from build123d import *

# Parameters (mm, degrees)
ESBO_O1_W                = 20
ESBO_O1_H                = 28
ESBO_O1_R                = 1.5
RESSALTO_EXTRUS_O1_DEPTH = 6
ESBO_O2_W                = 5
ESBO_O2_H                = 12
RESSALTO_EXTRUS_O2_START = -29
ESBO_O3_W                = 20
ESBO_O3_H                = 20
RESSALTO_EXTRUS_O2_DEPTH = 10
CORTE_EXTRUS_O1_DEPTH    = 28


with BuildPart() as part:
    # Esboço1 → Ressalto-extrusão1 (new body, symmetric)
    with BuildSketch(Plane.XY):
        Rectangle(ESBO_O1_W, ESBO_O1_H)
        with Locations((-7, 10)):
            Circle(ESBO_O1_R, mode=Mode.SUBTRACT)
        with Locations((7, 10)):
            Circle(ESBO_O1_R, mode=Mode.SUBTRACT)
    extrude(amount=RESSALTO_EXTRUS_O1_DEPTH, both=True)

    # Esboço2 → Revolução1 (revolve)
    with BuildSketch(Plane.XY):
        Polygon((3, -29), (3, -19), (3, -14), (0, -14), (0, -34), (0.75, -34), (3.5, -32), (3.5, -29), align=None)
        with Locations((2.5, 20)):
            Rectangle(ESBO_O2_W, ESBO_O2_H)
    revolve(axis=Axis((0, 0, 0), (0, -1, 0)))

    # Esboço3 → Ressalto-extrusão2 (add)
    with BuildSketch(Plane(origin=(0, 0, 0), x_dir=(1, 0, 0), z_dir=(0, 1, 0)).offset(RESSALTO_EXTRUS_O2_START)):
        with Locations((0, 4)):
            Rectangle(ESBO_O3_W, ESBO_O3_H)
    extrude(amount=RESSALTO_EXTRUS_O2_DEPTH)

    # Esboço4 → Corte-extrusão1 (cut)
    with BuildSketch(Plane(origin=(0, 14, 0), x_dir=(1, 0, 0), z_dir=(0, 1, 0))):
        with BuildLine():
            ThreePointArc((-10, 0), (-9.486832981, 3.16227766), (-8, 6))
            Line((-8, 6), (-10, 6))
            Line((-10, 6), (-10, 0))
        make_face()
        with BuildLine():
            ThreePointArc((-8, -6), (-9.486832981, -3.16227766), (-10, 0))
            Line((-10, 0), (-10, -6))
            Line((-10, -6), (-8, -6))
        make_face()
        with BuildLine():
            Line((10, -6), (10, 0))
            ThreePointArc((10, 0), (9.486832981, -3.16227766), (8, -6))
            Line((8, -6), (10, -6))
        make_face()
        with BuildLine():
            Line((10, 6), (8, 6))
            ThreePointArc((8, 6), (9.486832981, 3.16227766), (10, 0))
            Line((10, 0), (10, 6))
        make_face()
    extrude(amount=-CORTE_EXTRUS_O1_DEPTH, mode=Mode.SUBTRACT)


solid = part.part
Work out the finished part from the listing and answer in its coordinate system (mm). A direction names the side the tool comes from. Give positions to 0.01 mm unless a question says otherwise; leave off trailing zeros. Order: outer loops, then holes, each group sorted by start corner. A loop starts at its lowest first (then second) coordinate and runs counter-clockwise, first axis right, second up. Notation, with made-up numbers: M 59,18.25 L 115,18.25 A18 cw 115,44.25 Z; hole C -4.75,47.25 d2. An arc over 180 degrees is marked long. Return JSON: item names as keys, results as strings.
Q1. Each of these flat-tipped pins is pushed along its axis until it touches: pin 1 (1 mm diameter, centred on x = 4.5, y = -10.5, fed in from -Z); pin 2 (2.5 mm diameter, centred on x = -7, y = 10, fed in from -Z); pin 3 (1 mm diameter, centred on y = -17, z = 0, fed in from +X); pin 4 (4 mm diameter, centred on x = 2.5, z = -5, fed in from -Y). Where does it stop, or does it pass through?
Answer below:
{"pin 1": "stops at z = -6", "pin 2": "passes through", "pin 3": "stops at x = 3", "pin 4": "stops at y = -29"}
Q2. Which of the six approach directions +Z, -Z, +X, -X, +Y, -Y give full straight-line access (tool end or side, diameter ignored) to faces 4 (the face through (0, 0, -6)), 5 (the face through (-2, -14, -3)), 6 (the face through (-5, 14, -3))?
Answer below:
{"face 4": "-Z, +X, -X, +Y", "face 5": "none", "face 6": "+Y"}
Q3. Find section D-D, the plane y = 4. Write down the section's boundary in (x, z), and give its area (3 significant figures).
Answer below:
{"outline": "M -8,-6 L 8,-6 A10 ccw 8,6 L -8,6 A10 ccw Z", "area": "225 mm^2"}
Q4. Find section A-A, the plane x = 7. Write down the section's boundary in (y, z), and give its area (3 significant figures).
Answer below:
{"outline": "M -29,-14 L -19,-14 L -19,6 L -29,6 Z; M -14,-6 L 8.5,-6 L 8.5,6 L -14,6 Z; M 11.5,-6 L 14,-6 L 14,6 L 11.5,6 Z", "area": "500 mm^2"}
Q5. Find the intervals of material crossed by line 1 along Y through (x, z) = (-7, 2); line 2 along Y through (x, z) = (-4, -4.25); line 3 along X through (y, z) = (-12.5, 0.5), in increasing order. Write a range as [from, to].
Answer below:
{"line 1": "y = [-29, -19], [-14, 8.5], [11.5, 14]", "line 2": "y = [-29, -19], [-14, 14]", "line 3": "x = [-9.99, 9.99]"}
Q6. Find section B-B, the plane y = 10. Write down the section's boundary in (x, z).
Answer below:
{"outline": "M -8.5,-5.27 L -8.5,5.27 A10 ccw Z; M -5.5,-6 L 5.5,-6 L 5.5,6 L -5.5,6 Z; M 8.5,-5.27 A10 ccw 8.5,5.27 Z"}
Q7. The mould has two halves that part along Y. Classify faces 1 (the face through (-3, -16, 0)), 2 (the face through (-1.08, 20.08, -4.88)), 3 (the face through (0, -34, 0)): pulls with the +Y half, pulls with the -Y half, needs draft (parallel to the pull), parting line crosses it, or undercut.
Answer below:
{"face 1": "undercut", "face 2": "needs draft", "face 3": "pulls with the -Y half"}
Q8. Find section C-C, the plane x = 0. Write down the section's boundary in (y, z), and give its area (4 significant figures).
Answer below:
{"outline": "M -34,-0.75 L -32,-3.5 L -29,-3.5 L -29,-14 L -19,-14 L -19,-3 L -14,-3 L -14,-6 L 14,-6 L 14,-5 L 26,-5 L 26,5 L 14,5 L 14,6 L -14,6 L -14,3 L -19,3 L -19,6 L -29,6 L -29,3.5 L -32,3.5 L -34,0.75 Z", "area": "715.5 mm^2"}
